from build123d import *

# Parameters (mm, degrees)
SKETCH_1_R          = 12.5
SKETCH_1_R_2        = 11.5
EXTRUDE_1_DEPTH     = 17.5
SKETCH_2_R          = 12.5
SKETCH_2_R_2        = 11.5
SKETCH_1_3_R        = 11.5
CUT_EXTRUDE_2_DEPTH = 400


with BuildPart() as part:
    # 草圖1 → 填料-伸長1 (new, symmetric)
    with BuildSketch(Plane(origin=(0, 0, 0), x_dir=(1, 0, 0), z_dir=(0, 1, 0))):
        Circle(SKETCH_1_R)
        Circle(SKETCH_1_R_2, mode=Mode.SUBTRACT)
    extrude(amount=EXTRUDE_1_DEPTH, both=True)

    # 掃出1: sweep along a path in 草圖6
    with BuildLine(Plane.XY) as sweep_1_path:
        Line((0, 0), (155, 0))
        ThreePointArc((155, 0), (193.890872965, 16.109127035), (210, 55))
        Line((210, 55), (210, 260))
    # 草圖2 → 掃出1 (sweep)
    with BuildSketch(Plane(origin=(0, 0, 0), x_dir=(0, 0, -1), z_dir=(1, 0, 0))):
        Circle(SKETCH_2_R)
        Circle(SKETCH_2_R_2, mode=Mode.SUBTRACT)
    sweep(path=sweep_1_path.line)

    # 草圖1<3> → 除料-伸長2 (cut, symmetric)
    with BuildSketch(Plane(origin=(0, 0, 0), x_dir=(1, 0, 0), z_dir=(0, 1, 0))):
        Circle(SKETCH_1_3_R)
    extrude(amount=CUT_EXTRUDE_2_DEPTH, both=True, mode=Mode.SUBTRACT)


solid = part.part
Check sheet for the modelled part. Datum: model origin and axes. Units: mm. A direction names the side the tool comes from. Round coordinates to 2 decimals unless told otherwise and drop trailing zeros. Write each loop counter-clockwise with the first axis right and the second up, starting at its lowest first coordinate (ties: lowest second). Pieces come first, ordered by that corner, then holes. Notation, with made-up numbers: (-12, -6.5) -> (29, -6.5) arc R37 cw to (29, 30.5) -> close; hole circle Ø1 at (46.5, 87.5). An arc over 180 degrees is marked (long way). Answer as CSV lines item,"result". Start each with the question number.
1) Go/stop test with flat-tipped pins: P1, Ø10, axis at x = 21.5, z = 8.5, coming from the -Y side; P2, Ø4, axis at y = 69.5, z = -3.5, coming from the -X side; P3, Ø8, axis at y = 157.5, z = 5, coming from the +X side. Record where each tip stops, or that it passes through.
2) Material ranges on line 1 (X direction, y = 100, z = 0); line 2 (X direction, y = 6, z = 0); line 3 (Z direction, x = 0, y = 4.5), recorded low to high. Write a range as from..to.
3) Section check B-B on x = 135.5. Enter the section's corners in (y, z).
4) Section check C-C on y = 99.5. Enter the section's corners in (x, z), and give its area (3 significant figures).
5) Section check A-A on z = 0. Enter the section's corners in (x, y), and give its area (3 significant figures).
6) Tool access check on faces 4 (the cylindrical face through (78.585, 0.55, 12.488)), 5 (the flat face through (11, 17.5, 4)), 6 (the cylindrical face through (221.227, 158.935, 2.493)). Record the directions out of +Z, -Z, +X, -X, +Y, -Y that give a thin tool (end or side, any length) a straight path to the whole face; none if there is none.
7) Release check for a two-part mould opening along X. For faces 1 (the flat face through (206, 260, 11)), 2 (the cylindrical face through (197.606, 158.935, 1.627)), 3 (the cylindrical face through (81, 11.4, 1.5)) record: pulls with the +X half, pulls with the -X half, needs draft (parallel to the pull), parting line crosses it, or undercut.
8) Section check D-D on y = 0. State how many separate pieces and enclosed holes the cut face has, and give its area (3 significant figures).
Found:
1,P1,"stops at y = -12"
1,P2,"stops at x = 197.59"
1,P3,"stops at x = 222.46"
2,line 1,"x = 197.5..198.5, 221.5..222.5"
2,line 2,"x = -12.5..-11.5, 11.5..12.5, 199.96..201.42"
2,line 3,"z = -12.5..-11.5, 11.5..12.5"
3,outline,"circle Ø25 at (0, 0); hole circle Ø23 at (0, 0)"
4,outline,"circle Ø25 at (210, 0); hole circle Ø23 at (210, 0)"
4,area,"75.4 mm^2"
5,outline,"(-12.5, -17.5) -> (-11.5, -17.5) -> (-11.5, 17.5) -> (-12.5, 17.5) -> close; (11.5, -17.5) -> (12.5, -17.5) -> (12.5, -12.5) -> (155, -12.5) arc R67.5 ccw to (222.5, 55) -> (222.5, 260) -> (221.5, 260) -> (221.5, 55) arc R66.5 cw to (155, -11.5) -> (12.5, -11.5) -> (12.5, 11.5) -> (155, 11.5) arc R43.5 ccw to (198.5, 55) -> (198.5, 260) -> (197.5, 260) -> (197.5, 55) arc R42.5 cw to (155, 12.5) -> (12.5, 12.5) -> (12.5, 17.5) -> (11.5, 17.5) -> close"
5,area,"938 mm^2"
6,face 4,"none"
6,face 5,"+Z, -Z, -X, +Y"
6,face 6,"+Y"
7,face 1,"needs draft"
7,face 2,"parting line crosses it"
7,face 3,"undercut"
8,separate pieces,"1"
8,enclosed holes,"2"
8,area,"481 mm^2"
